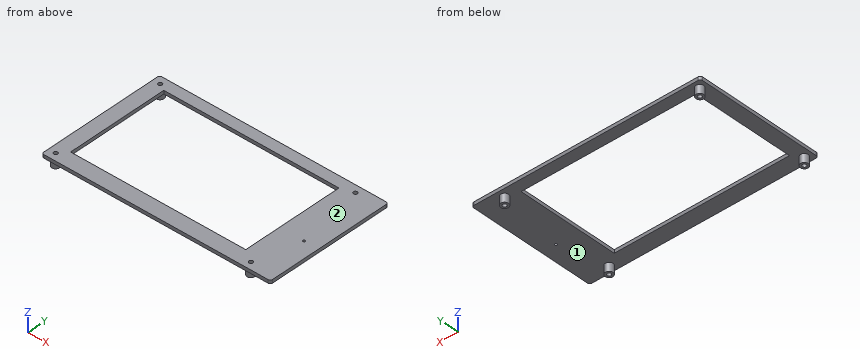
from build123d import *

# Parameters (mm, degrees)
F0_W      = 205
F0_H      = 115
F0_R      = 1.75
F0_W_2    = 157
F0_H_2    = 91
F1_DEPTH  = 3
F2_R      = 2
F3_DEPTH  = 25
F4_R      = 1
F5_DEPTH  = 25
F6_R      = 3.5
F7_DEPTH  = 7.5
F8_R      = 1.75
F9_DEPTH  = 25
F10_R     = 1.75
F11_DEPTH = 25
F12_R     = 1.75
F13_DEPTH = 25
F14_R     = 1.75
F15_DEPTH = 25


with BuildPart() as f1:
    # F0 (on Top) → F1 (new body)
    with BuildSketch(Plane.XY):
        with Locations((-16.301751, 5.736338)):
            Rectangle(F0_W, F0_H)
        with Locations((-112.301751, -45.263662)):
            Circle(F0_R, mode=Mode.SUBTRACT)
        with Locations((62.698249, -45.263662)):
            Circle(F0_R, mode=Mode.SUBTRACT)
        with Locations((-27.301751, 7.736338)):
            Rectangle(F0_W_2, F0_H_2, mode=Mode.SUBTRACT)
        with Locations((-112.301751, 56.736338)):
            Circle(F0_R, mode=Mode.SUBTRACT)
        with Locations((62.698249, 56.736338)):
            Circle(F0_R, mode=Mode.SUBTRACT)
    extrude(amount=F1_DEPTH)

    # F2
    f2_edges = [f1.edges().sort_by_distance(p)[0] for p in [
        (-118.801751, -51.763662, 1.5),
        (-118.801751, 63.236338, 1.5),
        (86.198249, -51.763662, 1.5),
        (86.198249, 63.236338, 1.5),
    ]]
    fillet(f2_edges, radius=F2_R)

    # F0 (on Top) → F3 (cut)
    with BuildSketch(Plane.XY):
        with Locations((-16.301751, 5.736338)):
            Rectangle(F0_W, F0_H)
        with Locations((-112.301751, -45.263662)):
            Circle(F0_R, mode=Mode.SUBTRACT)
        with Locations((62.698249, -45.263662)):
            Circle(F0_R, mode=Mode.SUBTRACT)
        with Locations((-27.301751, 7.736338)):
            Rectangle(F0_W_2, F0_H_2, mode=Mode.SUBTRACT)
        with Locations((-112.301751, 56.736338)):
            Circle(F0_R, mode=Mode.SUBTRACT)
        with Locations((62.698249, 56.736338)):
            Circle(F0_R, mode=Mode.SUBTRACT)
    extrude(amount=-F3_DEPTH, mode=Mode.SUBTRACT)

    # F4 (on face) → F5 (cut)
    with BuildSketch(Plane.XY.offset(3)):
        with Locations((73.198249, -4.763662)):
            Circle(F4_R)
    extrude(amount=-F5_DEPTH, mode=Mode.SUBTRACT)

    # F6 (on face) → F7 (join)
    with BuildSketch(Plane(origin=(0, 0, 0), x_dir=(1, 0, 0), z_dir=(0, 0, -1))):
        with Locations((-112.301751, 45.263662)):
            Circle(F6_R)
        with Locations((-112.301751, -56.736338)):
            Circle(F6_R)
        with Locations((62.698249, 45.263662)):
            Circle(F6_R)
        with Locations((62.698249, -56.736338)):
            Circle(F6_R)
    extrude(amount=F7_DEPTH)

    # F8 (on face) → F9 (cut)
    with BuildSketch(Plane(origin=(0, 0, -7.5), x_dir=(1, 0, 0), z_dir=(0, 0, -1))):
        with Locations((-112.301751, 45.263662)):
            Circle(F8_R)
    extrude(amount=-F9_DEPTH, mode=Mode.SUBTRACT)

    # F10 (on face) → F11 (cut)
    with BuildSketch(Plane(origin=(0, 0, -7.5), x_dir=(1, 0, 0), z_dir=(0, 0, -1))):
        with Locations((-112.301751, -56.736338)):
            Circle(F10_R)
    extrude(amount=-F11_DEPTH, mode=Mode.SUBTRACT)

    # F12 (on face) → F13 (cut)
    with BuildSketch(Plane(origin=(0, 0, -7.5), x_dir=(1, 0, 0), z_dir=(0, 0, -1))):
        with Locations((62.698249, -56.736338)):
            Circle(F12_R)
    extrude(amount=-F13_DEPTH, mode=Mode.SUBTRACT)

    # F14 (on face) → F15 (cut)
    with BuildSketch(Plane(origin=(0, 0, -7.5), x_dir=(1, 0, 0), z_dir=(0, 0, -1))):
        with Locations((62.698249, 45.263662)):
            Circle(F14_R)
    extrude(amount=-F15_DEPTH, mode=Mode.SUBTRACT)


solid = f1.part
The model under review builds one solid part; all positions refer to its coordinate system, in mm. Face numbers are marked on the shaded views. Coordinates: 2 decimals unless noted, no trailing zeros. Write each loop counter-clockwise with the first axis right and the second up, starting at its lowest first coordinate (ties: lowest second). Pieces come first, ordered by that corner, then holes. Notation, with made-up numbers: M 81,80 L 131,80 A14 cw 131,87 Z; hole C -36,-19 d9. An arc over 180 degrees is marked long. Put each result on its own line as item: value.
1) Add section A-A on y = 2.5. Give the boundary of the cut face in (x, z), then the cut area to 3 significant figures.
Computed:
outline: M -118.8,0 L -105.8,0 L -105.8,3 L -118.8,3 Z; M 51.2,0 L 86.2,0 L 86.2,3 L 51.2,3 Z
area: 144 mm2
2) Add section C-C on x = 9. Give the boundary of the cut face in (y, z).
Computed:
outline: M -51.76,0 L -37.76,0 L -37.76,3 L -51.76,3 Z; M 53.24,0 L 63.24,0 L 63.24,3 L 53.24,3 Z
3) Wall thickness on probe 1 along X at (y, z) = (-17, 2.5); probe 2 along Y at (x, z) = (-40, 1); probe 3 along X at (y, z) = (58, -6.5): over which ranges is each line inside the solid? List them lowest first. Write a range as [from, to].
Computed:
probe 1: x = [-118.8, -105.8], [51.2, 86.2]
probe 2: y = [-51.76, -37.76], [53.24, 63.24]
probe 3: x = [-115.57, -113.51], [-111.09, -109.04], [59.43, 61.49], [63.91, 65.96]
4) Add section B-B on z = -3.5. Give the boundary of the cut face in (x, y).
Computed:
outline: C -112.3,-45.26 d7; C -112.3,56.74 d7; C 62.7,-45.26 d7; C 62.7,56.74 d7; hole C -112.3,-45.26 d3.5; hole C -112.3,56.74 d3.5; hole C 62.7,-45.26 d3.5; hole C 62.7,56.74 d3.5
5) Draft analysis for pull direction X (two halves, no side actions). For the marked faces 1 and 2, state which applies: released by +X, released by -X, zero draft, split by the parting line, or undercut.
Computed:
face 1: undercut
face 2: zero draft
